Could you check a few things on this model? Use its own coordinates, in mm. A direction names the side the tool comes from. Round coordinates to 2 decimals unless told otherwise and drop trailing zeros. Loops run counter-clockwise (first coordinate to the right, second up) from the corner with the lowest first, then second, coordinate; pieces in that order, holes last. Notation, with made-up numbers: (-12.75, 60) -> (-6.75, 60) arc R23 ccw to (-6.75, 95) -> close; hole circle Ø10 at (41, -12.75). An arc over 180 degrees is marked (long way). Write each question's results on one line, items separated by ' | '.
from build123d import *

# Parameters (mm, degrees)
F0_W        = 21.5
F0_H        = 29
F1_DEPTH    = 15.7
F2_W        = 1.6
F2_H        = 0.8
F2_R        = 0.25
F2_W_2      = 0.8
F2_H_2      = 1.6
F3_DEPTH    = 3.75
F4_T1_DEPTH = 5.8
F4_T3_DEPTH = 5.8
F4_T5_DEPTH = 5.8


# Not quite as in the source:
# - a fillet or chamfer that OpenCascade refuses, or shapes differently, is made with other operations: its cross-section is extruded or revolved along the edge and cut away or added


with BuildPart() as f1:
    # F0 (on Top) → F1 (new body)
    with BuildSketch(Plane.XY):
        Rectangle(F0_W, F0_H)
    extrude(amount=F1_DEPTH)

    # F2 (on face) → F3 (join)
    with BuildSketch(Plane.XY):
        with Locations((8.63, 12.6)):
            Rectangle(F2_W, F2_H)
        with Locations((8.63, 4.98)):
            Rectangle(F2_W, F2_H)
        with Locations((-5.34, -10.26)):
            Circle(F2_R)
        with Locations((4.82, -10.26)):
            Circle(F2_R)
        with Locations((-9.15, 2.44)):
            Rectangle(F2_W_2, F2_H_2)
    extrude(amount=-F3_DEPTH)

    # F4: fillet of radius 1 on 6 edges, made by hand

    # F4_s2 → F4_t1 (cut)
    with BuildSketch(Plane.XZ.offset(-15.5)):
        with BuildLine():
            ThreePointArc((7.83, -2.75), (8.1228932188, -3.4571067812), (8.83, -3.75))
            Line((8.83, -3.75), (7.83, -3.75))
            Line((7.83, -3.75), (7.83, -2.75))
        make_face()
        with BuildLine():
            ThreePointArc((9.43, -2.75), (9.1371067812, -3.4571067812), (8.43, -3.75))
            Line((8.43, -3.75), (9.43, -3.75))
            Line((9.43, -3.75), (9.43, -2.75))
        make_face()
    extrude(amount=F4_T1_DEPTH, mode=Mode.SUBTRACT)

    # F4_s4 → F4_t3 (cut)
    with BuildSketch(Plane.XZ.offset(-7.88)):
        with BuildLine():
            ThreePointArc((7.83, -2.75), (8.1228932188, -3.4571067812), (8.83, -3.75))
            Line((8.83, -3.75), (7.83, -3.75))
            Line((7.83, -3.75), (7.83, -2.75))
        make_face()
        with BuildLine():
            ThreePointArc((9.43, -2.75), (9.1371067812, -3.4571067812), (8.43, -3.75))
            Line((8.43, -3.75), (9.43, -3.75))
            Line((9.43, -3.75), (9.43, -2.75))
        make_face()
    extrude(amount=F4_T3_DEPTH, mode=Mode.SUBTRACT)

    # F4_s6 → F4_t5 (cut)
    with BuildSketch(Plane.YZ.offset(-12.05)):
        with BuildLine():
            ThreePointArc((1.64, -2.75), (1.9328932188, -3.4571067812), (2.64, -3.75))
            Line((2.64, -3.75), (1.64, -3.75))
            Line((1.64, -3.75), (1.64, -2.75))
        make_face()
        with BuildLine():
            ThreePointArc((3.24, -2.75), (2.9471067812, -3.4571067812), (2.24, -3.75))
            Line((2.24, -3.75), (3.24, -3.75))
            Line((3.24, -3.75), (3.24, -2.75))
        make_face()
    extrude(amount=F4_T5_DEPTH, mode=Mode.SUBTRACT)


solid = f1.part
1) If we mould it in two halves opening along X, with no side actions, what happens to faces 1 (the flat face through (7.83, 5, -1)), 2 (the flat face through (-9, 1.64, -1)), 3 (the flat face through (9.43, 12.6, -1.4))? For each: released by +X, released by -X, zero draft, split by the parting line, or undercut.
Model answer:
face 1: released by -X | face 2: zero draft | face 3: released by +X
2) I want a section at A-A, the plane x = 1. Write out the boundary of the cut face in (y, z).
Model answer:
outline: (-14.5, 0) -> (14.5, 0) -> (14.5, 15.7) -> (-14.5, 15.7) -> close
3) I'm going to push flat-ended pins straight in: pin 1 (3 mm diameter, centred on x = -7.5, y = 5.5, fed in from -Z); pin 2 (1.3 mm diameter, centred on x = 8.5, z = -2, fed in from +Y); pin 3 (1.3 mm diameter, centred on y = 2.5, z = -2, fed in from +X); pin 4 (8 mm diameter, centred on x = -5, y = -10, fed in from -Z). Where does each tip first touch, or does it pass through?
Model answer:
pin 1: stops at z = 0 | pin 2: stops at y = 13 | pin 3: stops at x = -8.75 | pin 4: stops at z = -3.75
4) I need wall thicknesses on line 1 (Z direction, x = 2.75, y = 3.75); line 2 (X direction, y = 2, z = -0.5). Which ranges of each line are inside material? Lowest first, please.
Model answer:
line 1: z = 0 to 15.7 | line 2: x = -9.55 to -8.75
5) For faces 4 (the flat face through (9, 12.2, -2)), 5 (the flat face through (-8.75, 2, -2)), 6 (the flat face through (9, 4.58, -2)), 7 (the flat face through (7.83, 12.6, -1.4)), 8 (the flat face through (-9, 3.24, -1)), which set-ups out of +Z, -Z, +X, -X, +Y, -Y let a thin tool reach every point of the face, with its end or its side?
Model answer:
face 4: -Z, +X, -X | face 5: -Z, +X, +Y, -Y | face 6: -Z, +X, -X, -Y | face 7: -Z, -X, +Y, -Y | face 8: -Z, +X, -X, +Y
